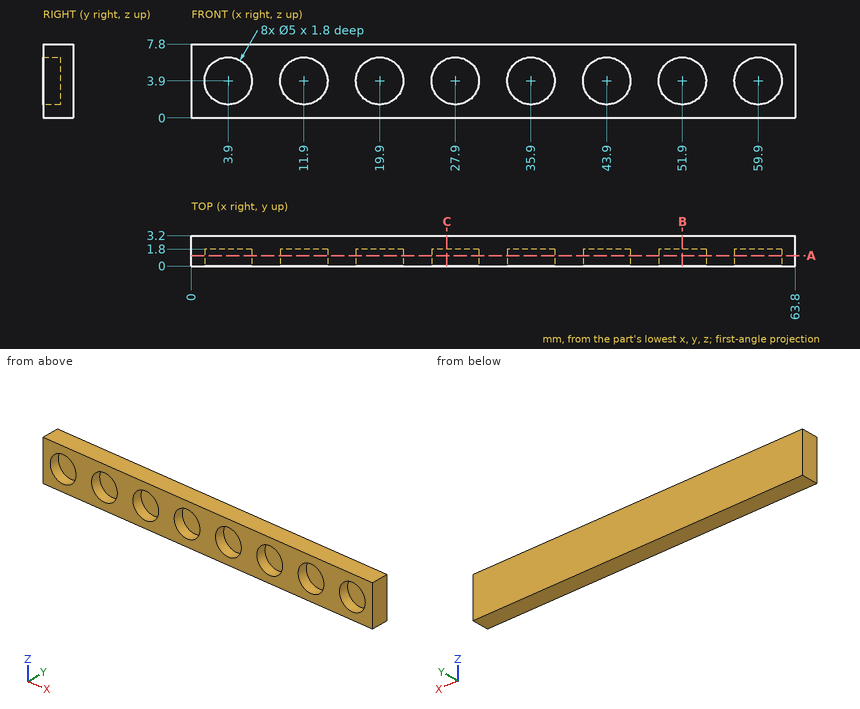
Can you work these out from the drawing? Everything is in mm from the part's minimum corner. Round coordinates to 2 decimals unless told otherwise and drop trailing zeros. Loops run counter-clockwise (first coordinate to the right, second up) from the corner with the lowest first, then second, coordinate; pieces in that order, holes last. Notation, with made-up numbers: (-7.5, 15.5) - (20.5, 15.5) arc R25 ccw to (20.5, 39.5) - close; hole circle Ø7 at (-4.5, -25.5). An arc over 180 degrees is marked (long way). One line per question, with ' | ' between items. Start each with the question number.
Q1. Will this pin go through, and if not, where does the flat tip stop? pin 1 (3 mm diameter, centred on x = 59.9, z = 3.9, fed in from -Y).
Q2. I want a section at A-A (y = 1.1). State how many separate pieces and enclosed holes the cut face has, then the cut area to 3 significant figures.
Q3. Please list where these lines run through material, in increasing order: line 1 (Z direction, x = 20, y = 0.5); line 2 (Y direction, x = 22, z = 4.75); line 3 (Z direction, x = 4.5, y = 1.2). Write a range as [from, to].
Q4. I want a section at B-B (x = 51.9). Write out the boundary of the cut face in (y, z).
Q5. I want a section at C-C (x = 27). Write out the boundary of the cut face in (y, z).
Response values:
1) pin 1: stops at y = 1.8
2) separate pieces: 1 | enclosed holes: 8 | area: 341 mm²
3) line 1: z = [0, 1.4], [6.4, 7.8] | line 2: y = [1.8, 3.2] | line 3: z = [0, 1.47], [6.33, 7.8]
4) outline: (0, 0) - (3.2, 0) - (3.2, 7.8) - (0, 7.8) - (0, 6.4) - (1.8, 6.4) - (1.8, 1.4) - (0, 1.4) - close
5) outline: (0, 0) - (3.2, 0) - (3.2, 7.8) - (0, 7.8) - (0, 6.23) - (1.8, 6.23) - (1.8, 1.57) - (0, 1.57) - close
